Work out the finished part from the listing and answer in its coordinate system (mm). Give positions to 0.01 mm unless a question says otherwise; leave off trailing zeros. Write each loop counter-clockwise with the first axis right and the second up, starting at its lowest first coordinate (ties: lowest second). Pieces come first, ordered by that corner, then holes. Notation, with made-up numbers: (64, 68) -> (106, 68) arc R9 cw to (106, 84) -> close; hole circle Ø6 at (69, -4.5). An arc over 180 degrees is marked (long way). Use a Markdown table: item, result. Add a question column.
Q1. Consider line 1 (Y direction, x = 15.25, z = 0.4); line 2 (Z direction, x = 9.5, y = -0.05); line 3 (Y direction, x = 5, z = -0.55). Determine where each line is inside the solid, lowest interval first.
Q2. Section A-A, the plane x = 12.25 is taken. Give the vertices of the cut face in (y, z), plus the area to 3 significant figures.
Q3. For a pull along Z with two mould halves and no side action, classify faces 1 (the face through (0, 0.4, 0.4)), 2 (the face through (8.16, 1.05, 0.33)), 3 (the face through (0.727, 0, 0)) as pulls with the +Z half, pulls with the -Z half, needs draft (parallel to the pull), parting line crosses it, or undercut.
Q4. Each of these flat-tipped pins is pushed along its axis until it touches: pin 1 Ø1 at (y, z) = (-0.5, 0.5) entering from -X; pin 2 Ø2 at (x, z) = (3.5, -0.5) entering from +Y; pin 3 Ø1 at (x, z) = (8.5, -1) entering from +Y. Where does it stop, or does it pass through?
Solid Edge part; units mm, degrees
sketch "Sketch1" plane through (0, 0, 0) normal (0, 0, 1) x (1, 0, 0)
  line L0 (0, 0) -> (0, 2.15)
  line L1 (0, 2.15) -> (0.25, 2.15)
  line L2 (0.25, 2.15) -> (1.0657, 1.3343)
  arc A0 (1.0657, 1.3343) -> (1.6314, 1.1) centre (1.6314, 1.9) ccw
  line L3 (1.6314, 1.1) -> (14.5, 1.1)
  line L4 (14.5, 1.1) -> (16, 0)
  line L5 (16, 0) -> (0, 0)
revolve "RevolvedProtrusion1" add sketch "Sketch1" angle 360 about axis through (20.3, 0, 0) along (-1, 0, 0)
cosmetic_thread "Thread_1" thread depth 12.4
sketch "Sketch2" plane through (0, 0, 0) normal (1, 0, 0) x (0, 1, 0)
  line L0 (0.2375, 0.95) -> (-0.2375, 0.95)
  line L1 (-0.2375, 0.95) -> (-0.1876, 0.38)
  line L2 (-0.1876, 0.38) -> (-0.2375, 0.2375)
  line L3 (-0.2375, 0.2375) -> (-0.38, 0.1876)
  line L4 (-0.38, 0.1876) -> (-0.95, 0.2375)
  line L5 (-0.95, 0.2375) -> (-0.95, -0.2375)
  line L6 (-0.95, -0.2375) -> (-0.38, -0.1876)
  line L7 (-0.38, -0.1876) -> (-0.2375, -0.2375)
  line L8 (-0.2375, -0.2375) -> (-0.1876, -0.38)
  line L9 (-0.1876, -0.38) -> (-0.2375, -0.95)
  line L10 (-0.2375, -0.95) -> (0.2375, -0.95)
  line L11 (0.2375, -0.95) -> (0.1876, -0.38)
  line L12 (0.1876, -0.38) -> (0.2375, -0.2375)
  line L13 (0.2375, -0.2375) -> (0.38, -0.1876)
  line L14 (0.38, -0.1876) -> (0.95, -0.2375)
  line L15 (0.95, -0.2375) -> (0.95, 0.2375)
  line L16 (0.95, 0.2375) -> (0.38, 0.1876)
  line L17 (0.38, 0.1876) -> (0.2375, 0.2375)
  line L18 (0.2375, 0.2375) -> (0.1876, 0.38)
  line L19 (0.1876, 0.38) -> (0.2375, 0.95)
extrude "ExtrudedCutout_1" cut sketch "Sketch2" along normal blind 0.7273
properties part number "bene_inox_212409-2,2X16"
Result set:
| question | item | result |
|---|---|---|
| 1 | line 1 | y = -0.38 to 0.38 |
| 1 | line 2 | z = -1.1 to 1.1 |
| 1 | line 3 | y = -0.95 to 0.95 |
| 2 | outline | circle Ø2.2 at (0, 0) |
| 2 | area | 3.80 mm2 |
| 3 | face 1 | needs draft |
| 3 | face 2 | parting line crosses it |
| 3 | face 3 | undercut |
| 4 | pin 1 | stops at x = 0 |
| 4 | pin 2 | stops at y = 1.1 |
| 4 | pin 3 | stops at y = 0.98 |
